from build123d import *

# Parameters (mm, degrees)
SKETCH2_W           = 39
SKETCH2_H           = 39
BOSS_EXTRUDE2_DEPTH = 6
SKETCH4_R           = 6.25
CUT_EXTRUDE2_DEPTH  = 6


with BuildPart() as part:
    # Sketch2 → Boss-Extrude2 (new body)
    with BuildSketch(Plane(origin=(0, 0, 0), x_dir=(1, 0, 0), z_dir=(0, 1, 0))):
        with Locations((-19.5, -19.5)):
            Rectangle(SKETCH2_W, SKETCH2_H)
    extrude(amount=-BOSS_EXTRUDE2_DEPTH)

    # Sketch4 → Cut-Extrude2 (cut)
    with BuildSketch(Plane.XZ.offset(6)):
        with Locations(Location((-19.5, 19.5, 0), (0, 0, 270))):
            Circle(SKETCH4_R)
    extrude(amount=-CUT_EXTRUDE2_DEPTH, mode=Mode.SUBTRACT)


solid = part.part
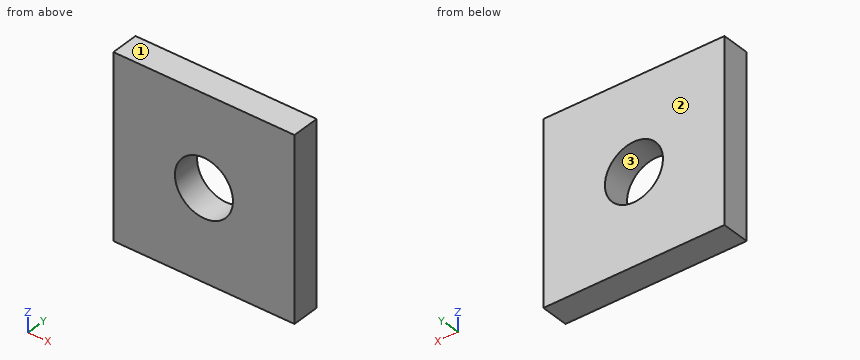
The listing builds one solid part. Answer for the finished solid, in the listing's coordinates (mm). Face numbers are marked on the shaded views. Coordinates: 2 decimals unless noted, no trailing zeros. Write each loop counter-clockwise with the first axis right and the second up, starting at its lowest first coordinate (ties: lowest second). Pieces come first, ordered by that corner, then holes. Notation, with made-up numbers: M -1.5,17.25 L 35.5,17.25 A27 cw 35.5,45.25 Z; hole C 71,80 d10. An arc over 180 degrees is marked long. Put each result on its own line as item: value. Start each with the question number.
1. A cutting plane is placed at C-C on y = -3.75. Write down the section's boundary in (x, z), then the cut area to 3 significant figures.
2. A flat-ended cylindrical pin translates along its axis: P1, Ø2, axis at x = -12, z = 32.5, coming from the +Y side. Find the tip coordinate at first contact, or state that the pin passes through.
3. A cutting plane is placed at B-B on z = 19.5. Write down the section's boundary in (x, y), then the cut area to 3 significant figures.
4. Consider line 1 (X direction, y = -3.8, z = 19.5); line 2 (Z direction, x = -15, y = -4.5); line 3 (X direction, y = -3.5, z = 16). Determine where each line is inside the solid, lowest interval first. Write a range as from..to.
5. For a pull along Z with two mould halves and no side action, classify the marked faces 1, 2 and 3 as pulls with the +Z half, pulls with the -Z half, needs draft (parallel to the pull), parting line crosses it, or undercut.
6. A cutting plane is placed at A-A on x = -19.5. Write down the section's boundary in (y, z).
Resolved:
1. outline: M -39,0 L 0,0 L 0,39 L -39,39 Z; hole C -19.5,19.5 d12.5
1. area: 1,400 mm2
2. P1: stops at y = 0
3. outline: M -39,-6 L -25.75,-6 L -25.75,0 L -39,0 Z; M -13.25,-6 L 0,-6 L 0,0 L -13.25,0 Z
3. area: 159 mm2
4. line 1: x = -39..-25.75, -13.25..0
4. line 2: z = 0..15.16, 23.84..39
4. line 3: x = -39..-24.68, -14.32..0
5. face 1: pulls with the +Z half
5. face 2: needs draft
5. face 3: undercut
6. outline: M -6,0 L 0,0 L 0,13.25 L -6,13.25 Z; M -6,25.75 L 0,25.75 L 0,39 L -6,39 Z
